Build history of the part. All positions in model axes, mm. Face numbers are marked on the shaded views. A direction names the side the tool comes from. Give positions to 0.01 mm unless a question says otherwise; leave off trailing zeros. Loops run counter-clockwise (first coordinate to the right, second up) from the corner with the lowest first, then second, coordinate; pieces in that order, holes last. Notation, with made-up numbers: (16.5, 86.25) - (59.5, 86.25) arc R15 cw to (59.5, 109.25) - close; hole circle Ø2 at (14.5, 72.5). An arc over 180 degrees is marked (long way). Return JSON: item names as keys, results as strings. Group by question number.
1) Slice it at D-D (y = 26). List the corners of the cut face in (x, z).
2) Slice it at B-B (y = -8.5). List the corners of the cut face in (x, z), and give its area (3 significant figures).
3) Mould opens along Y. For the marked faces 3, 4, 5 and 6 say: released by +Y, released by -Y, zero draft, split by the parting line, or undercut.
4) Slice it at C-C (z = 4). List the corners of the cut face in (x, y).
5) Drop flat-ended pins along their axis: pin 1 (3 mm diameter, centred on y = 11, z = 32, fed in from -X); pin 2 (2 mm diameter, centred on x = 15.5, z = 17, fed in from +Y); pin 3 (2 mm diameter, centred on x = -21, z = 12, fed in from +Y). Give the stop position or say it passes through.
6) 3-axis set-ups, long thin cutter, end or side, ignore diameter. For the marked faces 1 and 2: which of +Z, -Z, +X, -X, +Y, -Y reach the whole face in a straight line?
7) Slice it at A-A (x = -2.5). List the corners of the cut face in (y, z).
8) Drill centre lines: probe 1 along X at (y, z) = (-1.5, 14); probe 2 along Y at (x, z) = (20.5, 32.5); probe 3 along Y at (x, z) = (-13.5, 7). Where is each one in solid material? Low to high. Write a range as from..to.
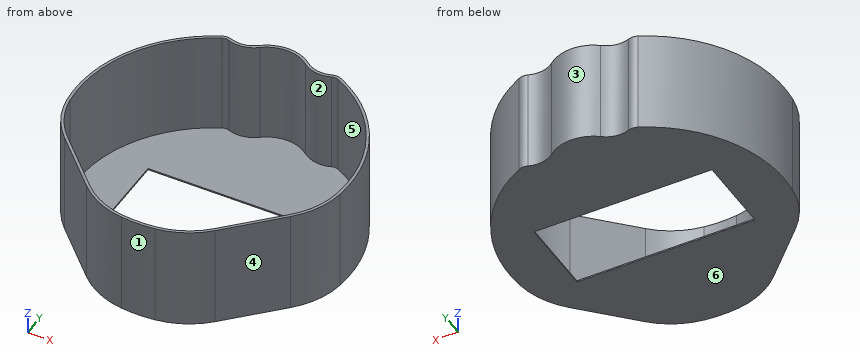
```python
from build123d import *

# Parameters (mm, degrees)
BOSS_EXTRUDE1_DEPTH = 37
CUT_EXTRUDE1_DEPTH  = 36.5
CUT_EXTRUDE2_REACH  = 80.556
SKETCH5_W           = 63.5
SKETCH5_H           = 28


with BuildPart() as part:
    # Sketch1 → Boss-Extrude1 (new body)
    with BuildSketch(Plane.XY):
        with BuildLine():
            Line((40.356535193, -22.947426174), (22.947426174, -40.356535193))
            ThreePointArc((22.947426174, -40.356535193), (15.156681171, -45.914203278), (5.981257322, -48.63357442))
            ThreePointArc((5.981257322, -48.63357442), (0, -49), (-5.981257322, -48.63357442))
            ThreePointArc((-5.981257322, -48.63357442), (-15.156681171, -45.914203278), (-22.947426174, -40.356535193))
            Line((-22.947426174, -40.356535193), (-40.356535193, -22.947426174))
            ThreePointArc((-40.356535193, -22.947426174), (-45.914203278, -15.156681171), (-48.63357442, -5.981257322))
            ThreePointArc((-48.63357442, -5.981257322), (-42.907888217, 23.662483572), (-20.892307913, 44.322809817))
            ThreePointArc((-20.892307913, 44.322809817), (-19.322951214, 44.702303901), (-17.73141344, 44.430451502))
            ThreePointArc((-17.73141344, 44.430451502), (-12.910393927, 43.910800792), (-8.488178405, 45.899839725))
            ThreePointArc((-8.488178405, 45.899839725), (0.386708758, 48.850803922), (9.16390657, 45.62084875))
            ThreePointArc((9.16390657, 45.62084875), (13.572775182, 43.625772556), (18.385878971, 44.128249799))
            ThreePointArc((18.385878971, 44.128249799), (20.002215513, 44.392928913), (21.589134046, 43.987603835))
            ThreePointArc((21.589134046, 43.987603835), (43.093258956, 23.323186587), (48.63357442, -5.981257322))
            ThreePointArc((48.63357442, -5.981257322), (45.914203278, -15.156681171), (40.356535193, -22.947426174))
        make_face()
    extrude(amount=BOSS_EXTRUDE1_DEPTH)

    # Sketch3 → Cut-Extrude1 (cut)
    with BuildSketch(Plane.XY.offset(37)):
        with BuildLine():
            Line((-39.649428412, -22.240319392), (-22.240319392, -39.649428412))
            ThreePointArc((-22.240319392, -39.649428412), (-14.718220769, -45.015452769), (-5.859190846, -47.641052493))
            ThreePointArc((-5.859190846, -47.641052493), (0, -48), (5.859190846, -47.641052493))
            ThreePointArc((5.859190846, -47.641052493), (14.718220769, -45.015452769), (22.240319392, -39.649428412))
            Line((22.240319392, -39.649428412), (39.649428412, -22.240319392))
            ThreePointArc((39.649428412, -22.240319392), (45.015452769, -14.718220769), (47.641052493, -5.859190846))
            ThreePointArc((47.641052493, -5.859190846), (42.213804691, 22.847203188), (21.148539474, 43.089897634))
            ThreePointArc((21.148539474, 43.089897634), (19.958350574, 43.393891443), (18.746098167, 43.195382107))
            ThreePointArc((18.746098167, 43.195382107), (13.413001918, 42.638618817), (8.52781313, 44.849236713))
            ThreePointArc((8.52781313, 44.849236713), (0.378047137, 47.850813988), (-7.865478644, 45.117238565))
            ThreePointArc((-7.865478644, 45.117238565), (-12.761098878, 42.921980343), (-18.095263428, 43.498993941))
            ThreePointArc((-18.095263428, 43.498993941), (-19.288916758, 43.702883241), (-20.465934283, 43.418262678))
            ThreePointArc((-20.465934283, 43.418262678), (-42.032217029, 23.179575744), (-47.641052493, -5.859190846))
            ThreePointArc((-47.641052493, -5.859190846), (-45.015452769, -14.718220769), (-39.649428412, -22.240319392))
        make_face()
    extrude(amount=-CUT_EXTRUDE1_DEPTH, mode=Mode.SUBTRACT)

    # Sketch5 → Cut-Extrude2 (cut, up to next)
    with BuildSketch(Plane(origin=(0, 0, 0), x_dir=(-1, 0, 0), z_dir=(0, 0, -1)), mode=Mode.PRIVATE) as cut_extrude2_sk1:
        with Locations((-0.5, 0.886817972)):
            Rectangle(SKETCH5_W, SKETCH5_H)
    cut_extrude2_tool1 = extrude(cut_extrude2_sk1.sketch, amount=-CUT_EXTRUDE2_REACH, mode=Mode.PRIVATE) & part.part
    add(cut_extrude2_tool1.solids().sort_by_distance((0.5, 0.886818, 0))[0], mode=Mode.SUBTRACT)


solid = part.part
```
Results:
{
 "1": {"outline": "(-41.53, 0) - (41.53, 0) - (41.53, 37) - (40.35, 37) - (40.35, 0.5) - (-40.35, 0.5) - (-40.35, 37) - (-41.53, 37) - close"},
 "2": {"outline": "(-48.21, 0) - (-31.25, 0) - (-31.25, 0.5) - (-47.19, 0.5) - (-47.19, 37) - (-48.21, 37) - close; (32.25, 0) - (48.21, 0) - (48.21, 37) - (47.19, 37) - (47.19, 0.5) - (32.25, 0.5) - close", "area": "91.2 mm2"},
 "3": {"face 3": "released by +Y", "face 4": "released by -Y", "face 5": "undercut", "face 6": "zero draft"},
 "4": {"outline": "(-48.63, -5.98) arc R29 ccw to (-40.36, -22.95) - (-22.95, -40.36) arc R29 ccw to (-5.98, -48.63) arc R49 ccw to (5.98, -48.63) arc R29 ccw to (22.95, -40.36) - (40.36, -22.95) arc R29 ccw to (48.63, -5.98) arc R49 ccw to (21.59, 43.99) arc R4 ccw to (18.39, 44.13) arc R9.26 cw to (9.16, 45.62) arc R14.15 ccw to (-8.49, 45.9) arc R9.26 cw to (-17.73, 44.43) arc R4 ccw to (-20.89, 44.32) arc R49 ccw to start; hole (-47.64, -5.86) arc R28 ccw to (-39.65, -22.24) - (-22.24, -39.65) arc R28 ccw to (-5.86, -47.64) arc R48 ccw to (5.86, -47.64) arc R28 ccw to (22.24, -39.65) - (39.65, -22.24) arc R28 ccw to (47.64, -5.86) arc R48 ccw to (21.15, 43.09) arc R3 ccw to (18.75, 43.2) arc R10.26 cw to (8.53, 44.85) arc R13.15 ccw to (-7.87, 45.12) arc R10.26 cw to (-18.1, 43.5) arc R3 ccw to (-20.47, 43.42) arc R48 ccw to start"},
 "5": {"pin 1": "x = -48.07", "pin 2": "y = 43.62", "pin 3": "y = 44.62"},
 "6": {"face 1": "+Z, -Z, -Y", "face 2": "+Z"},
 "7": {"outline": "(-48.94, 0) - (-13.11, 0) - (-13.11, 0.5) - (-47.93, 0.5) - (-47.93, 37) - (-48.94, 37) - close; (14.89, 0) - (48.6, 0) - (48.6, 37) - (47.58, 37) - (47.58, 0.5) - (14.89, 0.5) - close"},
 "8": {"probe 1": "-48.98..-47.98, 47.98..48.98", "probe 2": "-42.54..-41.25, 43.32..44.34", "probe 3": "-46.66..-45.57, 42.83..43.84"}
}
